from build123d import *

# Parameters (mm, degrees)
F0_W      = 1000
F0_H      = 500
F0_W_2    = 860
F0_H_2    = 360
F1_DEPTH  = 5
F2_R      = 6
F3_DEPTH  = 10
F5_R      = 6
F6_DEPTH  = 500
F8_DEPTH  = 30
F10_W     = 60
F10_H     = 140
F11_DEPTH = 10
F13_R     = 6
F14_DEPTH = 10
F17_R     = 6
F18_DEPTH = 908
F20_DEPTH = 40
F22_SIZE  = 10
F21_R     = 12.5
F23_DEPTH = 1


with BuildPart() as f1:
    # F0 (on Top) → F1 (new body, symmetric)
    with BuildSketch(Plane.XY):
        Rectangle(F0_W, F0_H)
        Rectangle(F0_W_2, F0_H_2, mode=Mode.SUBTRACT)
    extrude(amount=F1_DEPTH, both=True)

    # F2 (on face) → F3 (join)
    with BuildSketch(Plane.XZ.offset(250)):
        with BuildLine():
            ThreePointArc((-474, 41), (-481.7781745931, 37.7781745931), (-485, 30))
            Line((-485, 30), (-485, 15))
            Line((-485, 15), (-495, 15))
            Line((-495, 15), (-495, 5))
            Line((-495, 5), (-453, 5))
            Line((-453, 5), (-453, 15))
            Line((-453, 15), (-463, 15))
            Line((-463, 15), (-463, 30))
            ThreePointArc((-463, 30), (-466.2218254069, 37.7781745931), (-474, 41))
        make_face()
        with Locations((-474, 30)):
            Circle(F2_R, mode=Mode.SUBTRACT)
        with BuildLine():
            ThreePointArc((474, 41), (466.2218254069, 37.7781745931), (463, 30))
            Line((463, 30), (463, 15))
            Line((463, 15), (453, 15))
            Line((453, 15), (453, 5))
            Line((453, 5), (495, 5))
            Line((495, 5), (495, 15))
            Line((495, 15), (485, 15))
            Line((485, 15), (485, 30))
            ThreePointArc((485, 30), (481.7781745931, 37.7781745931), (474, 41))
        make_face()
        with Locations((474, 30)):
            Circle(F2_R, mode=Mode.SUBTRACT)
    extrude(amount=-F3_DEPTH)

    # F4: F1 across plane


with BuildPart() as f1_1:
    add(f1.part)
    add(f1.part.mirror(Plane.XZ))

    # F5 (on face) → F6 (join, through all)
    with BuildSketch(Plane.XZ.offset(250)):
        with Locations((-474, 30)):
            Circle(F5_R)
        with Locations((474, 30)):
            Circle(F5_R)
    extrude(amount=-F6_DEPTH)

    # F7 (on Front) → F8 (join, symmetric)
    with BuildSketch(Plane.XZ):
        with BuildLine():
            ThreePointArc((-474, 21), (-469.7722855411, 22.0547856886), (-466.5355339059, 24.9719043435))
            Line((-466.5355339059, 24.9719043435), (-461.5355339059, 24.9719043435))
            Line((-461.5355339059, 24.9719043435), (-458, 28.5074382495))
            Line((-458, 28.5074382495), (-458, 40))
            Line((-458, 40), (-474, 40))
            Line((-474, 40), (-490, 40))
            Line((-490, 40), (-490, 28.5074382495))
            Line((-490, 28.5074382495), (-486.4644660941, 24.9719043435))
            Line((-486.4644660941, 24.9719043435), (-481.4644660941, 24.9719043435))
            ThreePointArc((-481.4644660941, 24.9719043435), (-478.2277144589, 22.0547856886), (-474, 21))
        make_face()
    extrude(amount=F8_DEPTH, both=True)

    # F9: F1 across plane


with BuildPart() as f1_2:
    add(f1_1.part)
    add(f1_1.part.mirror(Plane.YZ))

    # F10 (on face) → F11 (join)
    with BuildSketch(Plane.XY.offset(40)):
        with Locations((-474, 0)):
            Rectangle(F10_W, F10_H)
    extrude(amount=F11_DEPTH)

    # F12: F1 across plane


with BuildPart() as f1_3:
    add(f1_2.part)
    add(f1_2.part.mirror(Plane.YZ))

    # F13 (on face) → F14 (join)
    with BuildSketch(Plane.YZ.offset(-444)):
        with BuildLine():
            Line((28, 60), (28, 50))
            Line((28, 50), (49, 50))
            Line((49, 50), (70, 50))
            Line((70, 50), (70, 60))
            Line((70, 60), (60, 60))
            Line((60, 60), (60, 75))
            ThreePointArc((60, 75), (56.7781745931, 82.7781745931), (49, 86))
            ThreePointArc((49, 86), (41.2218254069, 82.7781745931), (38, 75))
            Line((38, 75), (38, 60))
            Line((38, 60), (28, 60))
        make_face()
        with Locations((49, 75)):
            Circle(F13_R, mode=Mode.SUBTRACT)
    extrude(amount=-F14_DEPTH)

    # F15: F1 across plane


with BuildPart() as f1_4:
    add(f1_3.part)
    add(f1_3.part.mirror(Plane.XZ))

    # F16: F1 across plane


with BuildPart() as f1_5:
    add(f1_4.part)
    add(f1_4.part.mirror(Plane.YZ))

    # F17 (on face) → F18 (join, through all)
    with BuildSketch(Plane(origin=(-454, 0, 0), x_dir=(0, -1, 0), z_dir=(-1, 0, 0))):
        with Locations((-49, 75)):
            Circle(F17_R)
        with Locations((49, 75)):
            Circle(F17_R)
    extrude(amount=-F18_DEPTH)

    # F19 (on face) → F20 (join)
    with BuildSketch(Plane.XY.offset(50)):
        Polygon((-456.3223304703, -17.6776695297), (-491.6776695297, 17.6776695297), (-495.9203102168, 13.4350288425), (-460.5649711575, -21.9203102168), align=None)
    extrude(amount=F20_DEPTH)

    # F22
    f22_edges = [f1_5.edges().sort_by_distance(p)[0] for p in [
        (-458.443651, -19.79899, 90),
        (-493.79899, 15.556349, 90),
    ]]
    chamfer(f22_edges, length=F22_SIZE)

    # F21 (on face) → F23 (cut)
    with BuildSketch(Plane(origin=(-237, -237, 0), x_dir=(-0.7071067812, 0.7071067812, 0), z_dir=(0.7071067812, 0.7071067812, 0))):
        with Locations((335.1686142824, 70)):
            Circle(F21_R)
    extrude(amount=-F23_DEPTH, mode=Mode.SUBTRACT)


solid = f1_5.part
Can you work these out from the model? Positions are in its coordinate system, mm. A direction names the side the tool comes from. Round coordinates to 2 decimals unless told otherwise and drop trailing zeros. Write each loop counter-clockwise with the first axis right and the second up, starting at its lowest first coordinate (ties: lowest second). Pieces come first, ordered by that corner, then holes. Notation, with made-up numbers: (38, 38.5) -> (92, 38.5) arc R22 cw to (92, 63.5) -> close; hole circle Ø9 at (81, 82.5). An arc over 180 degrees is marked (long way). One line per question, with ' | ' between items. Start each with the question number.
1) On a 3-axis mill with a long thin cutter (end or side, diameter ignored), from which of +Z, -Z, +X, -X, +Y, -Y can I reach the whole of each face in a straight line? I mean faces 1 (the flat face through (-454, -49, 64)), 2 (the flat face through (-478, -30, 35)), 3 (the flat face through (454, -49, 64)), 4 (the flat face through (-7, -219, -5)). Say none if no direction works.
2) Suppose I cut it at C-C on y = -112. Write out the boundary of the cut face in (x, z), then the cut area to 3 significant figures.
3) I need wall thicknesses on line 1 (X direction, y = 53, z = 57.5); line 2 (X direction, y = -90, z = 31); line 3 (Z direction, x = -116.5, y = 201.5). Which ranges of each line are inside material? Lowest first, please. Write a range as [from, to].
4) Suppose I cut it at A-A on x = -247. Write out the boundary of the cut face in (y, z), then the cut area to 3 significant figures.
5) Suppose I cut it at B-B on y = 199.5. Write out the boundary of the cut face in (x, z).
6) I'm going to push flat-ended pins straight in: P1, Ø5, axis at y = -74, z = 25.5, coming from the +X side; P2, Ø5, axis at x = -447, y = 33, coming from the +Z side; P3, Ø12.5, axis at y = 7, z = 32.5, coming from the -X side. Where does each tip first touch, or does it pass through?
7) If we mould it in two halves opening along Y, with no side actions, what happens to faces 5 (the flat face through (-474, 240, 19)), 6 (the flat face through (-454, 49, 64))? For each: released by +Y, released by -Y, zero draft, split by the parting line, or undercut.
Return value:
1) face 1: +Z, -X, +Y, -Y | face 2: none | face 3: +Z, +X, +Y, -Y | face 4: -Z, +X, -X, +Y, -Y
2) outline: (-500, -5) -> (-430, -5) -> (-430, 5) -> (-500, 5) -> close; circle Ø12 at (-474, 30); (430, -5) -> (500, -5) -> (500, 5) -> (430, 5) -> close; circle Ø12 at (474, 30) | area: 1,630 mm2
3) line 1: x = [-454, -444], [444, 454] | line 2: x = [-479.92, -468.08], [468.08, 479.92] | line 3: z = [-5, 5]
4) outline: (-250, -5) -> (-180, -5) -> (-180, 5) -> (-250, 5) -> close; circle Ø12 at (-49, 75); circle Ø12 at (49, 75); (180, -5) -> (250, -5) -> (250, 5) -> (180, 5) -> close | area: 1,630 mm2
5) outline: (-500, -5) -> (500, -5) -> (500, 5) -> (-500, 5) -> close; circle Ø12 at (-474, 30); circle Ø12 at (474, 30)
6) P1: stops at x = 479.66 | P2: stops at z = 60 | P3: stops at x = -490
7) face 5: undercut | face 6: zero draft
